Source: CAD feature listing. Evaluate the final solid. Frame: model axes, mm. A direction names the side the tool comes from. Give positions to 0.01 mm unless a question says otherwise; leave off trailing zeros. Order: outer loops, then holes, each group sorted by start corner. A loop starts at its lowest first (then second) coordinate and runs counter-clockwise, first axis right, second up. Notation, with made-up numbers: M 70,9.5 L 116,9.5 A13 ccw 116,34.5 Z; hole C -37.75,15 d6. An arc over 180 degrees is marked long. Answer as a JSON object with one key per item and string values. Group by question number.
1. Set-up query: faces 1 (the flat face through (-235, -2, 3)), 2 (the flat face through (227.5, -2, -7.4)), 3 (the cylindrical face through (-231.302, -4.032, -6.324)). Return all of +Z, -Z, +X, -X, +Y, -Y with unobstructed straight access to the full face (end or side cutting, diameter ignored); none if empty.
2. Pin query (flat end, axial travel): P1, Ø2, axis at y = 0, z = 0.5, coming from the +X side. Return the tip coordinate at first contact, or that it passes through.
3. Section query A-A (x = -35). Output: boundary loops of the cut face in (y, z), plus the area to 3 significant figures.
4. Material intervals for L1, parallel to Z at x = -228.5, y = 0; L2, parallel to Z at x = -224.5, y = 0; L3, parallel to Z at x = 13, y = -0.75, sorted ascending. Write a range as [from, to].
from build123d import *


with BuildPart() as part:
    # Çizim1 → Döndür2 (revolve)
    with BuildSketch(Plane.XY, mode=Mode.PRIVATE) as d_nd_r2_sk:
        Polygon((-235, 0), (235, 0), (235, 7.5), (227.5, 7.5), (227.5, 9), (-227.5, 9), (-227.5, 7.5), (-235, 7.5), align=None)
    revolve(d_nd_r2_sk.sketch.rotate(Axis((-235, 0, 0), (1, 0, 0)), 180), axis=Axis((-235, 0, 0), (1, 0, 0)))

    # Çizim4 → M8 Dişli Delik3 (revolve, cut)
    with BuildSketch(Plane(origin=(-235, 0, 0), x_dir=(0, 0, 1), z_dir=(0, 1, 0))):
        Polygon((0, 0), (0, 24.292926105), (3.4, 22.25), (3.4, 0), align=None)
    m8_di_li_delik3 = revolve(axis=Axis((-241.35, 0, 0), (1, 0, 0)), mode=Mode.SUBTRACT)

    # Aynalama1: M8 Dişli Delik3 across plane
    add(m8_di_li_delik3.mirror(Plane(origin=(0, 0, 0), x_dir=(0, 0, 1), z_dir=(1, 0, 0))), mode=Mode.SUBTRACT)


solid = part.part
Answer sheet:
{
 "1": {"face 1": "+Z, -Z, -X, +Y, -Y", "face 2": "+X", "face 3": "-X"},
 "2": {"P1": "x = 211.61"},
 "3": {"outline": "C 0,0 d18", "area": "254 mm^2"},
 "4": {"L1": "[-7.5, -3.4], [3.4, 7.5]", "L2": "[-9, -3.4], [3.4, 9]", "L3": "[-8.97, 8.97]"}
}
